Can you work these out from the model? Positions are in its coordinate system, mm. Give positions to 0.01 mm unless a question says otherwise; leave off trailing zeros. Write each loop counter-clockwise with the first axis right and the second up, starting at its lowest first coordinate (ties: lowest second). Pieces come first, ordered by that corner, then holes. Notation, with made-up numbers: (80.25, 21) -> (89.25, 21) arc R20 ccw to (89.25, 43) -> close; hole circle Ø6 at (42, 34). An arc over 180 degrees is marked (long way). Answer as CSV lines item,"result". Start each with the question number.
1. I need wall thicknesses on line 1 (Z direction, x = 13, y = -9.5); line 2 (X direction, y = -1, z = -13); line 3 (X direction, y = -5, z = -12.5). Which ranges of each line are inside material? Lowest first, please. Write a range as [from, to].
2. I'm going to push a flat-ended pin straight in: P1, Ø4, axis at x = -92, y = -7, coming from the -Z side. Where does the tip first touch, or does it pass through?
3. If we section it at A-A on x = -63: Write out the boundary of the cut face in (y, z).
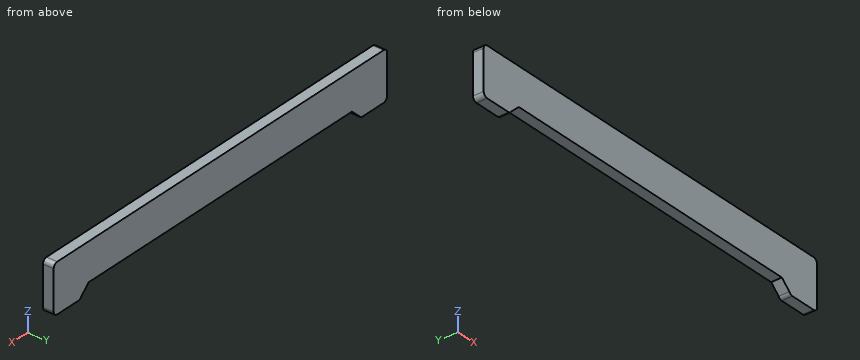
```python
from build123d import *

# Parameters (mm, degrees)
SKETCH_W     = 380
SKETCH_H     = 45
PAD_DEPTH    = 10
FILLET_R     = 4
SKETCH001_W  = 316
SKETCH001_H  = 14.743673
POCKET_DEPTH = 10
FILLET001_R  = 4
CHAMFER_SIZE = 8


with BuildPart() as part:
    # Sketch → Pad (new body)
    with BuildSketch(Plane.XZ):
        with Locations((0, 2.5)):
            Rectangle(SKETCH_W, SKETCH_H)
    extrude(amount=PAD_DEPTH)

    # Fillet
    fillet_edges = [part.edges().sort_by_distance(p)[0] for p in [
        (-190, -5, 25),
        (-190, -5, -20),
        (190, -5, -20),
        (190, -5, 25),
    ]]
    fillet(fillet_edges, radius=FILLET_R)

    # Sketch001 (on Face5 of Fillet) → Pocket (cut)
    with BuildSketch(Plane.XZ.offset(10)):
        with Locations((0, -17.294962)):
            Rectangle(SKETCH001_W, SKETCH001_H)
    extrude(amount=-POCKET_DEPTH, mode=Mode.SUBTRACT)

    # Fillet001
    fillet001_edges = [part.edges().sort_by_distance(p)[0] for p in [
        (-158, -5, -20),
        (158, -5, -20),
    ]]
    fillet(fillet001_edges, radius=FILLET001_R)

    # Chamfer
    chamfer_edges = [part.edges().sort_by_distance(p)[0] for p in [
        (-158, -5, -9.923126),
        (158, -5, -9.923126),
    ]]
    chamfer(chamfer_edges, length=CHAMFER_SIZE)


solid = part.part
```
Computed values:
1,line 1,"z = [-9.92, 25]"
1,line 2,"x = [-190, -153.27], [153.27, 190]"
1,line 3,"x = [-190, -152.74], [152.74, 190]"
2,P1,"stops at z = -9.92"
3,outline,"(-10, -9.92) -> (0, -9.92) -> (0, 25) -> (-10, 25) -> close"
